Autodesk Inventor part; units mm, degrees
ref_plane "YZ Plane" through (0, 0, 0) normal (1, 0, 0) x (0, 1, 0)
ref_plane "XZ Plane" through (0, 0, 0) normal (0, 1, 0) x (-1, 0, 0)
ref_plane "XY Plane" through (0, 0, 0) normal (0, 0, 1) x (1, 0, 0)
sketch "Sketch1" plane through (0, 0, 0) normal (0, 0, 1) x (1, 0, 0)
  line L0 (-42.4234, 22.9681) -> (-17.0234, 22.9681)
  line L1 (-17.0234, 22.9681) -> (-17.0234, -2.4319)
  line L2 (-17.0234, -2.4319) -> (-42.4234, -2.4319)
  line L3 (-42.4234, -2.4319) -> (-42.4234, 22.9681)
  point P0 (0, 0)
  dimension "d0" = 25.4
  dimension "d1" = 25.4
extrude "Extrusion1" add sketch "Sketch1" along normal blind 50.8
sketch "Sketch2" plane through (-17.0234, -2.4319, 0) normal (1, 0, 0) x (0, 0, -1)
  line L0 (-50.8, 22.86) -> (-50.8, 2.54)
  line L1 (-50.8, 2.54) -> (-55.88, 7.62)
  line L2 (-55.88, 7.62) -> (-76.2, 7.62)
  line L3 (-76.2, 7.62) -> (-76.2, 17.78)
  line L4 (-76.2, 17.78) -> (-55.88, 17.78)
  line L5 (-55.88, 17.78) -> (-50.8, 22.86)
  line L6 (-50.8, 0) -> (-50.8, 25.4)
  line L7 (0, 0) -> (-50.8, 0)
  point P0 (0, 2.4319)
  dimension "d4" = 25.4
  dimension "d5" = 20.32
  dimension "d6" = 5.08
  dimension "d7" = 5.08
  dimension "d8" = 5.08
  dimension "d9" = 5.08
  dimension "d10" = 0
  dimension "d11" = 2.54
extrude "Extrusion2" add sketch "Sketch2" against normal blind 25.4
sketch "Sketch3" plane through (-17.0234, -2.4319, 0) normal (1, 0, 0) x (0, 0, -1)
  line L0 (0, 20.4965) -> (0, 2.54)
  line L1 (0, 2.54) -> (5.08, 7.62)
  line L2 (5.08, 7.62) -> (25.4, 7.62)
  line L3 (25.4, 7.62) -> (25.4, 17.78)
  line L4 (25.4, 17.78) -> (5.08, 17.78)
  line L5 (5.08, 17.78) -> (0, 22.86)
  line L6 (0, 22.86) -> (0, 20.4965)
  line L7 (-55.88, 7.62) -> (-76.2, 7.62)
  line L8 (-76.2, 17.78) -> (-55.88, 17.78)
  line L9 (0, 25.4) -> (0, 0)
  line L10 (0, 0) -> (-50.8, 0)
  point P0 (0, 2.4319)
  dimension "d14" = 20.32
  dimension "d15" = 5.08
  dimension "d16" = 5.08
  dimension "d17" = 5.08
  dimension "d18" = 5.08
  dimension "d19" = 25.4
  dimension "d20" = 10.16
  dimension "d21" = 0
  dimension "d22" = 2.54
  dimension "d23" = 10.16
extrude "Extrusion3" add sketch "Sketch3" against normal blind 25.4
sketch "Sketch4" plane through (-17.0234, 5.1881, 76.2) normal (0, 0, 1) x (1, 0, 0)
  line L0 (0, 10.16) -> (-25.4, 10.16)
  line L1 (-25.4, 0) -> (-25.4, 10.16)
  point P0 (17.0234, -5.1881)
  point P1 (-12.7, 5.08)
  dimension "d26" = 5.08
  dimension "d27" = 12.7
hole "Hole1" at (-29.7234, 10.2681, 76.2) direction (0, 0, -1) diameter 6.477 end through all
sketch "Sketch5" plane through (-17.0234, 22.9681, 50.8) normal (1, 0, 0) x (0, 0, -1)
  line L0 (50.8, -25.4) -> (0, -25.4)
  point P0 (50.8, -22.9681)
  point P1 (12.7, -20.32)
  point P2 (38.1, -20.32)
  dimension "d35" = 5.08
  dimension "d36" = 5.08
  dimension "d37" = 12.7
  dimension "d38" = 12.7
hole "Hole2" at (-17.0234, 2.6481, 38.1) at (-17.0234, 2.6481, 12.7) direction (-1, 0, 0) diameter 4.9784 end through all
sketch "Sketch7" plane through (-17.0234, 22.9681, 50.8) normal (1, 0, 0) x (0, 0, -1)
  line L0 (-29.4216, -5.046) -> (-25.273, -5.046)
  line L1 (-25.273, -5.046) -> (-25.273, -20.1383)
  line L2 (-25.273, -20.1383) -> (-29.4216, -20.1383)
  line L3 (-29.4216, -20.1383) -> (-29.4216, -5.046)
  line L4 (-25.4, -17.78) -> (-25.4, -7.62)
  point P0 (50.8, -22.9681)
  dimension "d62" = 0.127
extrude "Extrusion4" cut sketch "Sketch7" against normal blind 50.8
sketch "Sketch8" plane through (-17.0234, -2.4319, 50.8) normal (1, 0, 0) x (0, 0, -1)
  line L0 (-27.9283, 21.8935) -> (-5.0883, 21.8935)
  line L1 (-5.0883, 21.8935) -> (-5.0883, 17.653)
  line L2 (-5.0883, 17.653) -> (-27.9283, 17.653)
  line L3 (-27.9283, 17.653) -> (-27.9283, 21.8935)
  line L4 (-25.273, 17.78) -> (-5.08, 17.78)
  line L5 (-26.1368, 7.747) -> (-5.0807, 7.747)
  line L6 (-5.0807, 7.747) -> (-5.0807, 5.4826)
  line L7 (-5.0807, 5.4826) -> (-26.1368, 5.4826)
  line L8 (-26.1368, 5.4826) -> (-26.1368, 7.747)
  line L9 (-5.08, 7.62) -> (-25.273, 7.62)
  point P0 (50.8, 2.4319)
  dimension "d65" = 0.127
  dimension "d66" = 0.127
extrude "Extrusion5" cut sketch "Sketch8" against normal blind 50.8
sketch "Sketch9" plane through (-42.4234, 22.9681, 0) normal (-1, 0, 0) x (0, 0, 1)
  line L0 (-28.1622, -4.7577) -> (-5.0787, -4.7577)
  line L1 (-5.0787, -4.7577) -> (-5.0787, -7.747)
  line L2 (-5.0787, -7.747) -> (-28.1622, -7.747)
  line L3 (-28.1622, -7.747) -> (-28.1622, -4.7577)
  line L4 (-27.0984, -17.653) -> (-5.0787, -17.653)
  line L5 (-5.0787, -17.653) -> (-5.0787, -20.2143)
  line L6 (-5.0787, -20.2143) -> (-27.0984, -20.2143)
  line L7 (-27.0984, -20.2143) -> (-27.0984, -17.653)
  line L8 (-29.1947, -5.6651) -> (-25.273, -5.6651)
  line L9 (-25.273, -5.6651) -> (-25.273, -18.8063)
  line L10 (-25.273, -18.8063) -> (-29.1947, -18.8063)
  line L11 (-29.1947, -18.8063) -> (-29.1947, -5.6651)
  line L12 (-25.4, -7.62) -> (-25.4, -17.78)
  line L13 (-5.08, -7.62) -> (-25.4, -7.62)
  line L14 (-25.4, -17.78) -> (-5.08, -17.78)
  point P0 (0, -22.9681)
  dimension "d69" = 0.127
  dimension "d70" = 0.127
  dimension "d71" = 0.127
extrude "Extrusion6" cut sketch "Sketch9" against normal blind 50.8
sketch "Sketch10" plane through (-42.4234, -2.4319, 0) normal (-1, 0, 0) x (0, 0, 1)
  line L0 (-2.7564, 0.127) -> (53.3126, 0.127)
  line L1 (53.3126, 0.127) -> (53.3126, -2.1248)
  line L2 (53.3126, -2.1248) -> (-2.7564, -2.1248)
  line L3 (-2.7564, -2.1248) -> (-2.7564, 0.127)
  line L4 (50.673, -3.7518) -> (52.4991, -3.7518)
  line L5 (52.4991, -3.7518) -> (52.4991, 2.4319)
  line L6 (52.4991, 2.4319) -> (50.673, 2.4319)
  line L7 (50.673, 2.4319) -> (50.673, -3.7518)
  line L8 (0.127, -3.5953) -> (-2.3183, -3.5953)
  line L9 (-2.3183, -3.5953) -> (-2.3183, 2.4319)
  line L10 (-2.3183, 2.4319) -> (0.127, 2.4319)
  line L11 (0.127, 2.4319) -> (0.127, -3.5953)
  line L12 (0, 0) -> (0, 2.54)
  line L13 (0, 0) -> (50.8, 0)
  line L14 (50.8, 2.54) -> (50.8, 0)
  point P0 (0, 2.4319)
  dimension "d74" = 0.127
  dimension "d75" = 0.127
  dimension "d76" = 0.127
extrude "Extrusion7" cut sketch "Sketch10" against normal blind 50.8
sketch "Sketch11" plane through (-42.4234, 22.9681, 0) normal (-1, 0, 0) x (0, 0, 1)
  line L0 (-3.471, 3.7894) -> (53.579, 3.7894)
  line L1 (53.579, 3.7894) -> (53.579, -1.27)
  line L2 (53.579, -1.27) -> (-3.471, -1.27)
  line L3 (-3.471, -1.27) -> (-3.471, 3.7894)
  line L4 (49.53, 5.7803) -> (53.579, 5.7803)
  line L5 (53.579, 5.7803) -> (53.579, -2.5925)
  line L6 (53.579, -2.5925) -> (49.53, -2.5925)
  line L7 (49.53, -2.5925) -> (49.53, 5.7803)
  line L8 (1.27, 6.2042) -> (-3.2289, 6.2042)
  line L9 (-3.2289, 6.2042) -> (-3.2289, -2.5925)
  line L10 (-3.2289, -2.5925) -> (1.27, -2.5925)
  line L11 (1.27, -2.5925) -> (1.27, 6.2042)
  line L12 (0, -2.54) -> (0, 0)
  line L13 (0, 0) -> (50.8, 0)
  line L14 (50.8, 0) -> (50.8, -2.54)
  point P0 (0, -22.9681)
  dimension "d79" = 1.27
  dimension "d80" = 1.27
  dimension "d81" = 1.27
extrude "Extrusion8" cut sketch "Sketch11" against normal blind 50.8
sketch "Sketch13" plane through (-42.4234, 5.3151, 76.073) normal (-1, 0, 0) x (0, 0, 1)
  line L0 (-81.1517, 0) -> (-81.1517, -0.1283)
  line L1 (-81.1517, 0) -> (-81.1517, -0.1283)
  line L2 (-81.1517, -0.1283) -> (-76.073, -5.207)
  line L3 (-81.1517, -0.1283) -> (-76.073, -5.207)
  line L4 (-76.073, -5.3151) -> (-75.946, -5.3151)
  line L5 (-76.073, -5.3151) -> (-75.946, -5.3151)
  line L6 (-75.946, -5.3151) -> (-75.946, -5.2062)
  line L7 (-76.073, -5.3151) -> (-76.073, -5.207)
  line L8 (-76.073, -5.3151) -> (-76.073, -5.207)
  line L9 (-81.1517, 0) -> (-75.946, -5.2062)
extrude "Extrusion9" cut sketch "Sketch13" against normal blind 50.8
sketch "Sketch14" plane through (-42.4234, 5.3151, 76.073) normal (-1, 0, 0) x (0, 0, 1)
  line L0 (-81.1517, 9.906) -> (-81.1517, 10.0343)
  line L1 (-81.1517, 9.906) -> (-81.1517, 10.0343)
  line L2 (-76.1255, 15.0605) -> (-74.803, 15.0605)
  line L3 (-81.1517, 10.0343) -> (-76.1255, 15.0605)
  line L4 (-81.1517, 10.0343) -> (-76.1255, 15.0605)
  line L5 (-76.1255, 15.0605) -> (-74.803, 15.0605)
  line L6 (-74.803, 15.0605) -> (-74.803, 16.383)
  line L7 (-74.803, 15.0605) -> (-81.1517, 9.906)
  point P0 (-76.073, -5.3151)
extrude "Extrusion10" cut sketch "Sketch14" against normal blind 50.8
sketch "Sketch16" plane through (-42.4234, 5.3151, 76.073) normal (-1, 0, 0) x (0, 0, 1)
  line L0 (-26.543, 15.0605) -> (-26.543, 16.383)
  line L1 (-20.193, 10.033) -> (-25.2205, 15.0605)
  line L2 (-26.543, 15.0605) -> (-25.2205, 15.0605)
  line L3 (-20.1847, 9.906) -> (-20.1847, 10.033)
  line L4 (-25.2205, 15.0605) -> (-20.1847, 10.033)
  line L5 (-26.543, 15.0605) -> (-20.1847, 9.906)
  line L6 (0, 9.906) -> (-20.1847, 9.906)
  line L7 (-20.1847, 9.906) -> (-20.1847, 10.033)
  point P0 (-76.073, -5.3151)
extrude "Extrusion11" cut sketch "Sketch16" against normal blind 50.8
sketch "Sketch18" plane through (-42.4234, 5.3151, 76.073) normal (-1, 0, 0) x (0, 0, 1)
  line L0 (-20.1923, 0) -> (-20.1923, -0.127)
  line L1 (-20.1923, 0) -> (-25.5398, -5.3151)
  line L2 (-25.5398, -5.3151) -> (-25.1146, -5.3151)
  line L3 (-25.1146, -5.3151) -> (-20.1923, -0.127)
  point P0 (-76.073, -5.3151)
extrude "Extrusion12" cut sketch "Sketch18" against normal blind 50.8
properties part number "SliderSlider"
The listing builds one solid part. Answer for the finished solid, in the listing's coordinates (mm). A direction names the side the tool comes from. Coordinates: 2 decimals unless noted, no trailing zeros. Loops run counter-clockwise (first coordinate to the right, second up) from the corner with the lowest first, then second, coordinate; pieces in that order, holes last. Notation, with made-up numbers: (86, 38) -> (105, 38) arc R30 ccw to (105, 71) -> close; hole circle Ø2 at (-10.75, -12.5). An arc over 180 degrees is marked (long way). Return JSON: item names as keys, results as strings. Group by question number.
(1) A cutting plane is placed at D-D on z = -2.5. Write down the section's boundary in (x, y), and give its area (3 significant figures).
(2) Find the intervals of material crossed by probe 1 along Z at (x, y) = (-30.25, 3.5); probe 2 along Z at (x, y) = (-30.25, -0.5); probe 3 along Y at (x, z) = (-20.5, 64), in increasing order. Write a range as from..to.
(3) A cutting plane is placed at C-C on x = -32. Write down the section's boundary in (y, z), and give its area (3 significant figures).
(4) Given pin 1 Ø1.8 at (x, y) = (-31.5, -1) entering from +Z; pin 2 Ø3 at (x, z) = (-29, 51) entering from -Y; pin 3 Ø10 at (x, z) = (-36, -19) entering from +Y; pin 4 Ø8 at (x, z) = (-23, -5.5) entering from +Y, each flat-ended and moving along its own axis, determine where each tip first touches the part or whether it passes through.
(5) Determine the mould class of faces 5 (the flat face through (-30, -1, 50.673)), 6 (the cylindrical face through (-29.901, 1.9, 10.326)), 7 (the cylindrical face through (-32.934, 10.69, 24.691)) for opening direction Z: released by +Z, released by -Z, zero draft, split by the parting line, or undercut.
(6) Which of the six approach directions +Z, -Z, +X, -X, +Y, -Y give full straight-line access (tool end or side, diameter ignored) to faces 1 (the flat face through (-30, 15.221, 66)), 2 (the flat face through (-30, 5.315, 66)), 3 (the flat face through (-30, 5.315, -15)), 4 (the flat face through (-30, 15.221, -15))?
(7) A cutting plane is placed at B-B on y = 9.75. Write down the section's boundary in (x, z), and give its area (3 significant figures).
(8) A cutting plane is placed at A-A on z = 38.5. Write down the section's boundary in (x, y).
The answers:
{
 "1": {"outline": "(-42.42, 2.74) -> (-17.02, 2.74) -> (-17.02, 17.31) -> (-42.42, 17.31) -> close; hole circle Ø6.48 at (-29.72, 10.27)", "area": "337 mm^2"},
 "2": {"probe 1": "z = -3.26..10.36, 15.04..35.76, 40.44..54.05", "probe 2": "z = 0.13..50.67", "probe 3": "y = 5.32..15.22"},
 "3": {"outline": "(-2.3, 0.13) -> (0.11, 0.13) -> (5.32, -5.08) -> (5.32, -25.27) -> (7.96, -25.27) -> (7.96, 76.07) -> (5.32, 76.07) -> (5.32, 55.88) -> (0, 50.53) -> (0, 50.67) -> (-2.3, 50.67) -> close; (12.57, -25.27) -> (15.22, -25.27) -> (15.22, -5.08) -> (20.38, 1.27) -> (21.7, 1.27) -> (21.7, 49.53) -> (20.38, 49.53) -> (15.22, 55.89) -> (15.22, 76.07) -> (12.57, 76.07) -> close; hole circle Ø4.98 at (2.65, 12.7); hole circle Ø4.98 at (2.65, 38.1)", "area": "1,260 mm^2"},
 "4": {"pin 1": "stops at z = 50.67", "pin 2": "stops at y = -2.3", "pin 3": "stops at y = 15.22", "pin 4": "stops at y = 18.13"},
 "5": {"face 5": "released by +Z", "face 6": "undercut", "face 7": "zero draft"},
 "6": {"face 1": "+Z, +X, -X, +Y", "face 2": "+Z, +X, -X, -Y", "face 3": "-Z, +X, -X, -Y", "face 4": "-Z, +X, -X, +Y"},
 "7": {"outline": "(-42.42, -25.27) -> (-32.92, -25.27) -> (-32.92, 76.07) -> (-42.42, 76.07) -> close; (-26.53, -25.27) -> (-17.02, -25.27) -> (-17.02, 76.07) -> (-26.53, 76.07) -> close", "area": "1,930 mm^2"},
 "8": {"outline": "(-42.42, -2.3) -> (-17.02, -2.3) -> (-17.02, 0.19) -> (-42.42, 0.19) -> close; (-42.42, 5.1) -> (-17.02, 5.1) -> (-17.02, 21.7) -> (-42.42, 21.7) -> close; hole circle Ø6.48 at (-29.72, 10.27)"}
}
